Geometry check sheet. Reference: drawing and pictorial views, mm from the part's lowest x, y, z. A direction names the side the tool comes from. Round coordinates to 2 decimals unless told otherwise and drop trailing zeros. Loops run counter-clockwise (first coordinate to the right, second up) from the corner with the lowest first, then second, coordinate; pieces in that order, holes last. Notation, with made-up numbers: (-20.75, 38) - (33.25, 38) arc R28 ccw to (33.25, 64) - close; hole circle Ø1 at (28.5, 49.5). An arc over 180 degrees is marked (long way). Put each result on its own line as item: value. Start each with the question number.
Item 1: Section check B-B, the plane z = 31. Record the cut outline in (x, y), and give its area (3 significant figures).
Item 2: Section check C-C, the plane x = 119. Record the cut outline in (y, z), and give its area (3 significant figures).
Item 3: Tool access check on the marked faces 1 and 2. Record the directions out of +Z, -Z, +X, -X, +Y, -Y that give a thin tool (end or side, any length) a straight path to the whole face; none if there is none.
Item 4: Gauge pin test, flat ends, axial feed: pin 1 Ø1 at (y, z) = (13, 46.5) entering from +X; pin 2 Ø8 at (x, y) = (87, 83.5) entering from +Z. Record the tip position at first contact, or that the pin passes through.
Item 5: Section check D-D, the plane y = 78. Record the cut outline in (x, z), and give its area (3 significant figures).
Item 6: Material ranges on line 1 along Z through (x, y) = (97.5, 44.5); line 2 along X through (y, z) = (12, 65); line 3 along Y through (x, z) = (34.5, 73), recorded low to high.
Item 7: Section check A-A, the plane y = 50.8. Record the cut outline in (x, z).
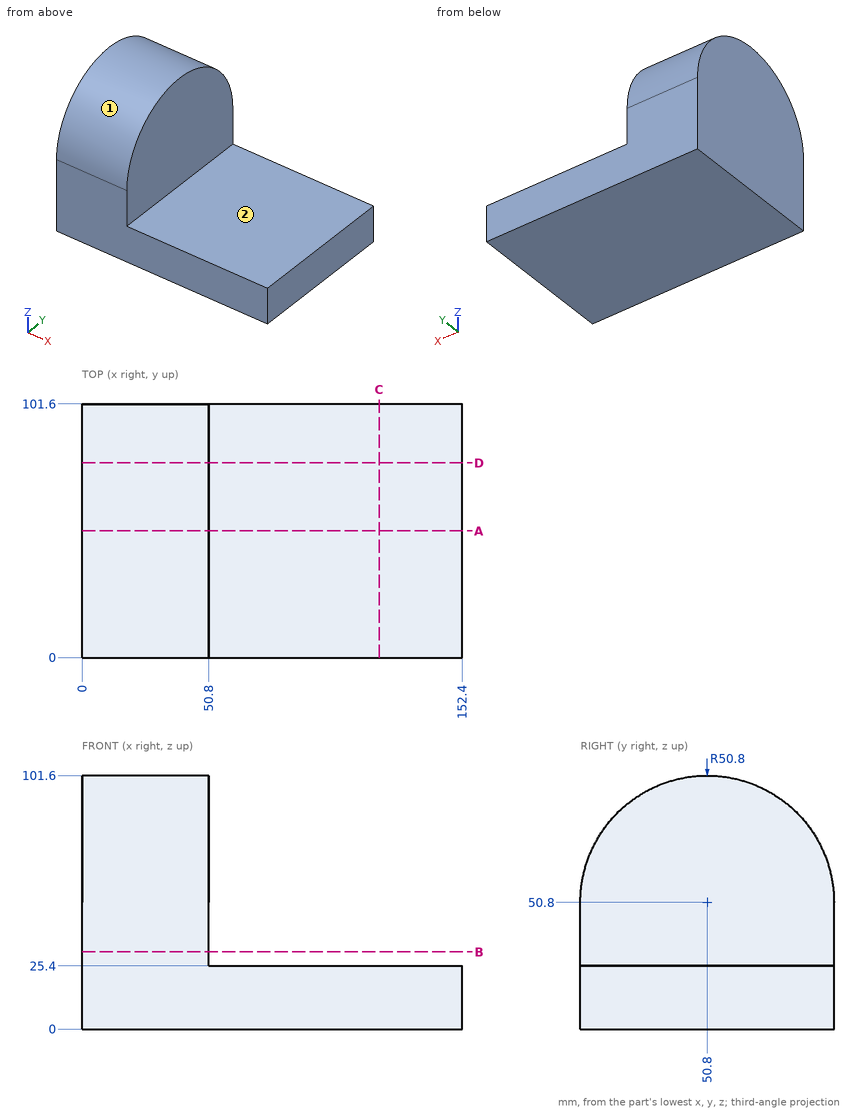
Check result:
1. outline: (0, 0) - (50.8, 0) - (50.8, 101.6) - (0, 101.6) - close
1. area: 5,160 mm²
2. outline: (0, 0) - (101.6, 0) - (101.6, 25.4) - (0, 25.4) - close
2. area: 2,580 mm²
3. face 1: +Z, +X, -X
3. face 2: +Z, +X, +Y, -Y
4. pin 1: x = 50.8
4. pin 2: z = 25.4
5. outline: (0, 0) - (152.4, 0) - (152.4, 25.4) - (50.8, 25.4) - (50.8, 93.7) - (0, 93.7) - close
5. area: 7,340 mm²
6. line 1: 0 to 25.4
6. line 2: 0 to 50.8
6. line 3: 5.11 to 96.49
7. outline: (0, 0) - (152.4, 0) - (152.4, 25.4) - (50.8, 25.4) - (50.8, 101.6) - (0, 101.6) - close
